Model file for the job. Use its own axes, mm. Face numbers are marked on the shaded views. A direction names the side the tool comes from. Round coordinates to 2 decimals unless told otherwise and drop trailing zeros. Order: outer loops, then holes, each group sorted by start corner. A loop starts at its lowest first (then second) coordinate and runs counter-clockwise, first axis right, second up. Notation, with made-up numbers: (28.5, 47) - (38.5, 47) arc R20 ccw to (38.5, 55) - close; hole circle Ø2 at (62.5, -8). An arc over 180 degrees is marked (long way). Use one line per item in the form item = value.
from build123d import *

# Parameters (mm, degrees)
SKETCH_1_W          = 42
SKETCH_1_H          = 42
EXTRUDE_1_DEPTH     = 5
CHAMFER_1_SIZE      = 5.5
SKETCH_2_R          = 1.5
CUT_EXTRUDE_1_DEPTH = 5
SKETCH_3_R          = 18
EXTRUDE_2_DEPTH     = 27.5
SKETCH_4_R          = 1.5
CUT_EXTRUDE_2_DEPTH = 4
SKETCH_6_R          = 11
EXTRUDE_3_DEPTH     = 2
SKETCH_7_R          = 4
EXTRUDE_4_DEPTH     = 18.5
SKETCH_8_R          = 11
CUT_EXTRUDE_3_DEPTH = 3
SKETCH_9_R          = 8
CUT_EXTRUDE_4_DEPTH = 10
CUT_EXTRUDE_START   = -15
CUT_EXTRUDE_5_DEPTH = 15
SKETCH_12_R         = 2.8
CUT_EXTRUDE_6_DEPTH = 3


with BuildPart() as part:
    # 草图1 → 凸台-拉伸1 (new body)
    with BuildSketch(Plane(origin=(0, 0, 0), x_dir=(1, 0, 0), z_dir=(0, 1, 0))):
        Rectangle(SKETCH_1_W, SKETCH_1_H)
    extrude(amount=EXTRUDE_1_DEPTH)

    # 倒角1
    chamfer_1_edges = [part.edges().sort_by_distance(p)[0] for p in [
        (21, 2.5, 21),
        (-21, 2.5, 21),
        (-21, 2.5, -21),
        (21, 2.5, -21),
    ]]
    chamfer(chamfer_1_edges, length=CHAMFER_1_SIZE)

    # 草图2 → 切除-拉伸1 (cut)
    with BuildSketch(Plane.XZ):
        with Locations(Location((-15.5, 15.5, 0), (0, 0, 270))):
            Circle(SKETCH_2_R)
        with Locations(Location((15.5, 15.5, 0), (0, 0, 270))):
            Circle(SKETCH_2_R)
        with Locations(Location((15.5, -15.5, 0), (0, 0, 270))):
            Circle(SKETCH_2_R)
        with Locations(Location((-15.5, -15.5, 0), (0, 0, 270))):
            Circle(SKETCH_2_R)
    extrude(amount=-CUT_EXTRUDE_1_DEPTH, mode=Mode.SUBTRACT)

    # 草图3 → 凸台-拉伸2 (add)
    with BuildSketch(Plane(origin=(0, 5, 0), x_dir=(1, 0, 0), z_dir=(0, 1, 0))):
        with Locations(Location((0, 0, 0), (0, 0, 270))):
            Circle(SKETCH_3_R)
    extrude(amount=EXTRUDE_2_DEPTH)

    # 草图4 → 切除-拉伸2 (cut)
    with BuildSketch(Plane(origin=(0, 32.5, 0), x_dir=(1, 0, 0), z_dir=(0, 1, 0))):
        with Locations(Location((-9.899494937, 9.899494937, 0), (0, 0, 270))):
            Circle(SKETCH_4_R)
        with Locations(Location((9.899494937, 9.899494937, 0), (0, 0, 270))):
            Circle(SKETCH_4_R)
        with Locations(Location((9.899494937, -9.899494937, 0), (0, 0, 270))):
            Circle(SKETCH_4_R)
        with Locations(Location((-9.899494937, -9.899494937, 0), (0, 0, 270))):
            Circle(SKETCH_4_R)
    extrude(amount=-CUT_EXTRUDE_2_DEPTH, mode=Mode.SUBTRACT)

    # 草图6 → 凸台-拉伸3 (add)
    with BuildSketch(Plane(origin=(0, 32.5, 0), x_dir=(1, 0, 0), z_dir=(0, 1, 0))):
        with Locations(Location((0, 0, 0), (0, 0, 270))):
            Circle(SKETCH_6_R)
    extrude(amount=EXTRUDE_3_DEPTH)

    # 草图7 → 凸台-拉伸4 (add)
    with BuildSketch(Plane(origin=(0, 34.5, 0), x_dir=(1, 0, 0), z_dir=(0, 1, 0))):
        with Locations(Location((0, 0, 0), (0, 0, 270))):
            Circle(SKETCH_7_R)
    extrude(amount=EXTRUDE_4_DEPTH)

    # 草图8 → 切除-拉伸3 (cut)
    with BuildSketch(Plane.XZ):
        with Locations(Location((0, 0, 0), (0, 0, 90))):
            Circle(SKETCH_8_R)
    extrude(amount=-CUT_EXTRUDE_3_DEPTH, mode=Mode.SUBTRACT)

    # 草图9 → 切除-拉伸4 (cut)
    with BuildSketch(Plane.XZ.offset(-3)):
        with Locations(Location((0, 0, 0), (0, 0, 270))):
            Circle(SKETCH_9_R)
    extrude(amount=-CUT_EXTRUDE_4_DEPTH, mode=Mode.SUBTRACT)

    # 草图11 → 切除-拉伸5 (cut)
    with BuildSketch(Plane(origin=(0, 53, 0), x_dir=(1, 0, 0), z_dir=(0, 1, 0)).offset(CUT_EXTRUDE_START)):
        with BuildLine():
            Line((-1.914185744, -3.512248986), (-1.914185744, 3.512248986))
            ThreePointArc((-1.914185744, 3.512248986), (-4, 0), (-1.914185744, -3.512248986))
        make_face()
    extrude(amount=CUT_EXTRUDE_5_DEPTH, mode=Mode.SUBTRACT)

    # 草图12 → 切除-拉伸6 (cut)
    with BuildSketch(Plane(origin=(0, 5, 0), x_dir=(1, 0, 0), z_dir=(0, 1, 0))):
        with Locations(Location((-15.5, 15.5, 0), (0, 0, 270))):
            Circle(SKETCH_12_R)
        with Locations(Location((15.5, 15.5, 0), (0, 0, 270))):
            Circle(SKETCH_12_R)
        with Locations(Location((-15.5, -15.5, 0), (0, 0, 270))):
            Circle(SKETCH_12_R)
        with Locations(Location((15.5, -15.5, 0), (0, 0, 270))):
            Circle(SKETCH_12_R)
    extrude(amount=-CUT_EXTRUDE_6_DEPTH, mode=Mode.SUBTRACT)


solid = part.part
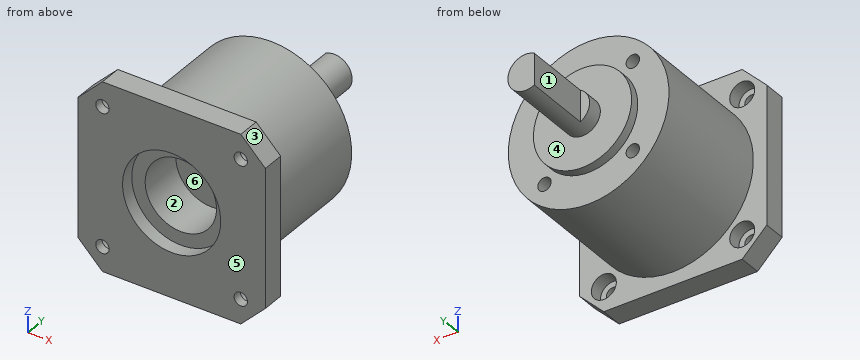
(1) Pull direction X, two halves, no side cores. Call the marked faces 1, 2 and 3: released by +X, released by -X, zero draft, split by the parting line, or undercut.
Report:
face_1 = released by -X
face_2 = undercut
face_3 = released by +X
(2) Tool access for the marked faces 4, 5 and 6: list every direction of +Z, -Z, +X, -X, +Y, -Y with a clear straight run to the whole face (end or side of a thin tool).
Report:
face_4 = +Y
face_5 = +Z, -Z, +X, -X, -Y
face_6 = -Y
(3) Slice it at D-D on y = 40.5. Give the cut face in (x, z).
Report:
outline = (-1.91, -3.51) arc R4 ccw (long way) to (-1.91, 3.51) - close
(4) Slice it at A-A on x = 0. Give the cut face in (y, z), then the cut area to 3 significant figures.
Report:
outline = (0, -21) - (5, -21) - (5, -18) - (32.5, -18) - (32.5, -11) - (34.5, -11) - (34.5, -4) - (53, -4) - (53, 4) - (34.5, 4) - (34.5, 11) - (32.5, 11) - (32.5, 18) - (5, 18) - (5, 21) - (0, 21) - (0, 11) - (3, 11) - (3, 8) - (13, 8) - (13, -8) - (3, -8) - (3, -11) - (0, -11) - close
area = 1,170 mm2
(5) Probe probe 1 along X at (y, z) = (2.6, -15.5); probe 2 along X at (y, z) = (0.4, -15.5); probe 3 along X at (y, z) = (1, 0). List the from-to ranges inside material, lowest first. Write a range as [from, to].
Report:
probe_1 = [-21, -18.3], [-12.7, 12.7], [18.3, 21]
probe_2 = [-21, -17], [-14, 14], [17, 21]
probe_3 = [-21, -11], [11, 21]
(6) Slice it at B-B on y = 10. Give the cut face in (x, z), then the cut area to 3 significant figures.
Report:
outline = circle Ø36 at (0, 0); hole circle Ø16 at (0, 0)
area = 817 mm2
(7) Pin check, flat tips, straight feed: pin 1 (5 mm diameter, centred on y = 24.5, z = 9.5, fed in from +X); pin 2 (12 mm diameter, centred on x = 10.5, z = -13, fed in from +Y); pin 3 (10 mm diameter, centred on y = 24, z = -4.5, fed in from +X). Stop position of each tip, or through.
Report:
pin_1 = 16.58
pin_2 = 34.5
pin_3 = 18
(8) Slice it at C-C on z = 0. Give the cut face in (x, y), then the cut area to 3 significant figures.
Report:
outline = (-21, 0) - (-11, 0) - (-11, 3) - (-8, 3) - (-8, 13) - (8, 13) - (8, 3) - (11, 3) - (11, 0) - (21, 0) - (21, 5) - (18, 5) - (18, 32.5) - (11, 32.5) - (11, 34.5) - (4, 34.5) - (4, 53) - (-1.91, 53) - (-1.91, 38) - (-4, 38) - (-4, 34.5) - (-11, 34.5) - (-11, 32.5) - (-18, 32.5) - (-18, 5) - (-21, 5) - close
area = 1,130 mm2
